Can you work these out from the model? Positions are in its coordinate system, mm. A direction names the side the tool comes from. Give positions to 0.01 mm unless a question says otherwise; leave off trailing zeros. Loops run counter-clockwise (first coordinate to the right, second up) from the corner with the lowest first, then second, coordinate; pieces in that order, holes last. Notation, with made-up numbers: (80, 64.5) - (118, 64.5) arc R17 cw to (118, 82.5) - close; hole circle Ø5 at (17.5, -18.5). An arc over 180 degrees is marked (long way). Write item = value, one per line.
from build123d import *

# Parameters (mm, degrees)
F1_DEPTH = 1
F3_DEPTH = 1.8
F4_DEPTH = 1


with BuildPart() as f1:
    # F0 (on Top) → F1 (new body)
    with BuildSketch(Plane.XY):
        with BuildLine():
            ThreePointArc((-10.9, 13.9), (-13.0213203436, 13.0213203436), (-13.9, 10.9))
            Line((-13.9, 10.9), (-13.9, -10.9))
            ThreePointArc((-13.9, -10.9), (-13.0213203436, -13.0213203436), (-10.9, -13.9))
            Line((-10.9, -13.9), (10.9, -13.9))
            ThreePointArc((10.9, -13.9), (13.0213203436, -13.0213203436), (13.9, -10.9))
            Line((13.9, -10.9), (13.9, 10.9))
            ThreePointArc((13.9, 10.9), (13.0213203436, 13.0213203436), (10.9, 13.9))
            Line((10.9, 13.9), (-10.9, 13.9))
        make_face()
        with BuildLine():
            Line((-13.1, -0.5), (-0.5, -0.5))
            Line((-0.5, -0.5), (-0.5, -13.1))
            Line((-0.5, -13.1), (-10.9, -13.1))
            ThreePointArc((-10.9, -13.1), (-12.4556349186, -12.4556349186), (-13.1, -10.9))
            Line((-13.1, -10.9), (-13.1, -0.5))
        make_face(mode=Mode.SUBTRACT)
        with BuildLine():
            Line((10.9, -13.1), (0.5, -13.1))
            Line((0.5, -13.1), (0.5, -0.5))
            Line((0.5, -0.5), (13.1, -0.5))
            Line((13.1, -0.5), (13.1, -10.9))
            ThreePointArc((13.1, -10.9), (12.4556349186, -12.4556349186), (10.9, -13.1))
        make_face(mode=Mode.SUBTRACT)
        with BuildLine():
            Line((-10.9, 13.1), (-0.5, 13.1))
            Line((-0.5, 13.1), (-0.5, 0.5))
            Line((-0.5, 0.5), (-13.1, 0.5))
            Line((-13.1, 0.5), (-13.1, 10.9))
            ThreePointArc((-13.1, 10.9), (-12.4556349186, 12.4556349186), (-10.9, 13.1))
        make_face(mode=Mode.SUBTRACT)
        with BuildLine():
            Line((13.1, 10.9), (13.1, 0.5))
            Line((13.1, 0.5), (0.5, 0.5))
            Line((0.5, 0.5), (0.5, 13.1))
            Line((0.5, 13.1), (10.9, 13.1))
            ThreePointArc((10.9, 13.1), (12.4556349186, 12.4556349186), (13.1, 10.9))
        make_face(mode=Mode.SUBTRACT)
    extrude(amount=F1_DEPTH)

    # F2 (on face) → F3 (join)
    with BuildSketch(Plane.XY.offset(1)):
        Polygon((-2.6832024986, 2.5549852797), (-11.1835549314, 2.4956311428), (-8.4767530422, 0.5), (-0.5, 0.5), (-0.5, 9.1179095817), align=None)
        Polygon((-0.5, 0.5), (-8.4767530422, 0.5), (-7.1203892177, -0.5), (-0.5, -0.5), (-0.5, -6.061026872), (0, -5.7030628772), (0.5, -6.061026872), (0.5, -0.5), (7.1203892177, -0.5), (8.4767530422, 0.5), (0.5, 0.5), (0.5, 9.1179095817), (0, 10.6209594147), (-0.5, 9.1179095817), align=None)
        Polygon((2.6832024986, 2.5549852797), (0.5, 9.1179095817), (0.5, 0.5), (8.4767530422, 0.5), (11.1835549314, 2.4956311428), align=None)
        Polygon((0.5, -0.5), (0.5, -6.061026872), (6.9118170627, -10.651426171), (4.3415128415, -2.548769162), (7.1203892177, -0.5), align=None)
        Polygon((-0.5, -0.5), (-7.1203892177, -0.5), (-4.3415128415, -2.548769162), (-6.9118170627, -10.651426171), (-0.5, -6.061026872), align=None)
    extrude(amount=F3_DEPTH)

    # F4 (add): faces of the model
    f4_faces = [f1.faces().sort_by_distance(p)[0] for p in [
        (-4.0960108107, 2.4354750497, 1),
        (-3.3222149953, -4.5114296876, 1),
        (3.3222149953, -4.5114296876, 1),
        (4.0960108107, 2.4354750497, 1),
    ]]
    extrude(f4_faces, amount=F4_DEPTH)


solid = f1.part
Q1. We'd pull the mould along Y, two halves only. Please class faces 3 (the flat face through (0.5, 11.1, 0.5)), 4 (the cylindrical face through (13, -13.04, 0.49)), 5 (the flat face through (0.2, 13.9, 0.5)), 6 (the flat face through (13.9, -0.2, 0.5)): released by +Y, released by -Y, zero draft, split by the parting line, or undercut.
Output:
face_3 = undercut
face_4 = released by -Y
face_5 = released by +Y
face_6 = zero draft
Q2. Imagine slicing it at A-A, the plane x = 4. Write out the boundary of the cut face in (y, z), then the cut area to 3 significant figures.
Output:
outline = (-13.9, 0) - (-13.1, 0) - (-13.1, 1) - (-13.9, 1) - close; (-8.57, 0) - (2.55, 0) - (2.55, 2.8) - (-8.57, 2.8) - close; (13.1, 0) - (13.9, 0) - (13.9, 1) - (13.1, 1) - close
area = 32.7 mm2
Q3. Imagine slicing it at B-B, the plane y = -11.25. Write out the boundary of the cut face in (x, z), then the cut area to 3 significant figures.
Output:
outline = (-13.88, 0) - (-13.07, 0) - (-13.07, 1) - (-13.88, 1) - close; (-0.5, 0) - (0.5, 0) - (0.5, 1) - (-0.5, 1) - close; (13.07, 0) - (13.88, 0) - (13.88, 1) - (13.07, 1) - close
area = 2.62 mm2
Q4. For pin 1 (5 mm diameter, centred on x = 8.5, y = 6, fed in from +Z); pin 2 (0.8 mm diameter, centred on y = 12, z = 0.5, fed in from -X); pin 3 (0.8 mm diameter, centred on x = 11.5, z = 0.5, fed in from +Y); pin 4 (1.5 mm diameter, centred on x = -11, z = 2, fed in from -Y), each with a flat end and sliding along its axis, tell me the tip position at first contact or that it passes through.
Output:
pin_1 = through
pin_2 = -13.82
pin_3 = 13.89
pin_4 = 1.81
Q5. Which directions (+Z, -Z, +X, -X, +Y, -Y) give clear straight access to the entire face, cutting with the end or side of a thin tool? Please do faces 1 (the flat face through (0, 0, 2.8)), 2 (the cylindrical face through (12.44, 12.47, 0.49)).
Output:
face_1 = +Z, +X, -X, +Y, -Y
face_2 = +Z, -Z
Q6. Imagine slicing it at D-D, the plane z = 2.05. Write out the boundary of the cut face in (x, y), then the cut area to 3 significant figures.
Output:
outline = (-11.18, 2.5) - (-4.34, -2.55) - (-6.91, -10.65) - (0, -5.7) - (6.91, -10.65) - (4.34, -2.55) - (11.18, 2.5) - (2.68, 2.55) - (0, 10.62) - (-2.68, 2.55) - close
area = 158 mm2
Q7. I need wall thicknesses on L1, parallel to X at y = -11, z = 0.75; L2, parallel to Y at x = -8, z = 0.75; L3, parallel to Y at x = -10.5, z = 0.6. Which ranges of each line are inside material? Lowest first, please.
Output:
L1 = -13.9 to -13.1, -0.5 to 0.5, 13.1 to 13.9
L2 = -13.9 to -13.1, -0.5 to 2.52, 13.1 to 13.9
L3 = -13.9 to -13.1, -0.5 to 0.5, 1.99 to 2.5, 13.1 to 13.9
Q8. Imagine slicing it at C-C, the plane z = 0.45. Give the number of separate pieces and of enclosed holes in the cut face, then the cut area to 3 significant figures.
Output:
separate_pieces = 1
enclosed_holes = 4
area = 262 mm2
